from build123d import *

# Parameters (mm, degrees)
F1_DEPTH = 40.2336
F0_R     = 10.16
F2_DEPTH = 15.7734
F3_R     = 3.302


with BuildPart() as f1:
    # F0 (on Front) → F1 (new body)
    with BuildSketch(Plane.XZ):
        with BuildLine():
            ThreePointArc((-46.7830288695, 26.6589681412), (-51.5056559342, 28.027918724), (-56.3930534915, 28.5669708617))
            Line((-56.3930534915, 28.5669708617), (-46.7830288695, 26.6589681412))
        make_face()
        with BuildLine():
            Line((-45.9697033865, -26.3306877774), (-57.2444129947, -28.5744701634))
            ThreePointArc((-57.2444129947, -28.5744701634), (-51.4930580564, -28.0254145609), (-45.9697033865, -26.3306877774))
        make_face()
        with BuildLine():
            Line((-46.7830288695, 26.6589681412), (-56.3930534915, 28.5669708617))
            ThreePointArc((-56.3930534915, 28.5669708617), (-85.6422307581, 0.4256962659), (-57.2444129947, -28.5744701634))
            Line((-57.2444129947, -28.5744701634), (-45.9697033865, -26.3306877774))
            ThreePointArc((-45.9697033865, -26.3306877774), (-33.2614425676, -15.8007621125), (-28.4954018406, 0))
            ThreePointArc((-28.4954018406, 0), (-33.506740117, 16.1642961856), (-46.7830288695, 26.6589681412))
        make_face()
        with BuildLine():
            ThreePointArc((-47.01702871, -10.1519626155), (-71.3571450466, -0.1470537858), (-47.2281253638, 10.3567490075))
            Line((-47.2281253638, 10.3567490075), (-38.5411018406, 10.3567490075))
            Line((-38.5411018406, 10.3567490075), (-38.5411018406, -10.1519626155))
            Line((-38.5411018406, -10.1519626155), (-47.01702871, -10.1519626155))
        make_face(mode=Mode.SUBTRACT)
    extrude(amount=F1_DEPTH)

    # F0 (on Front) → F2 (join)
    with BuildSketch(Plane.XZ):
        with BuildLine():
            Line((12.9274923096, 14.8038646076), (-46.7830288695, 26.6589681412))
            ThreePointArc((-46.7830288695, 26.6589681412), (-33.506740117, 16.1642961856), (-28.4954018406, 0))
            ThreePointArc((-28.4954018406, 0), (-33.2614425676, -15.8007621125), (-45.9697033865, -26.3306877774))
            Line((-45.9697033865, -26.3306877774), (12.9274923096, -14.6095441843))
            ThreePointArc((12.9274923096, -14.6095441843), (19.8690099187, 0.0971602116), (12.9274923096, 14.8038646076))
        make_face()
        with Locations((-3.0954018406, 0)):
            Circle(F0_R, mode=Mode.SUBTRACT)
    extrude(amount=F2_DEPTH)

    # F3
    f3_edges = [f1.edges().sort_by_distance(p)[0] for p in [
        (-57.74775, -40.2336, -28.566971),
    ]]
    fillet(f3_edges, radius=F3_R)


solid = f1.part
Geometry: final body of the model. Coordinates: model frame, mm. A direction names the side the tool comes from. Give positions to 0.01 mm unless a question says otherwise; leave off trailing zeros. Order: outer loops, then holes, each group sorted by start corner. A loop starts at its lowest first (then second) coordinate and runs counter-clockwise, first axis right, second up. Notation, with made-up numbers: (-23.75, 69.25) -> (2.25, 69.25) arc R18 ccw to (2.25, 94.25) -> close; hole circle Ø1 at (14.25, 29). An arc over 180 degrees is marked (long way). Answer as a JSON object with one key per item and string values.
Q1. Section A-A (y = -12). State how many separate pieces and enclosed holes the cut face has, plus the area to 3 significant figures.
Entries:
{"separate pieces": "1", "enclosed holes": "2", "area": "3,380 mm^2"}
Q2. Material intervals for probe 1 along X at (y, z) = (-28, 0); probe 2 along X at (y, z) = (-10, -4); probe 3 along Z at (x, y) = (-57, -35), sorted ascending.
Entries:
{"probe 1": "x = -85.65 to -71.36, -38.54 to -28.5", "probe 2": "x = -85.36 to -70.79, -38.54 to -12.43, 6.24 to 19.42", "probe 3": "z = -28.57 to -14.29, 14.29 to 28.57"}
Q3. Draft query along X for faces 3 (the flat face through (-38.541, -20, 0)), 4 (the flat face through (-14, -15.773, 1)), 5 (the flat face through (-16.93, -7.78, -20.55)). Return one class per face: released by +X, released by -X, zero draft, split by the parting line, or undercut.
Entries:
{"face 3": "undercut", "face 4": "zero draft", "face 5": "released by +X"}
Q4. First-contact query: pin 1 (8 mm diameter, centred on y = -16.5, z = 6.5, fed in from +X); pin 2 (9.5 mm diameter, centred on x = -44.5, y = -15.5, fed in from -Z); pin 3 (10 mm diameter, centred on x = -24.5, y = -10.5, fed in from +Z). Flat tips, straight axial feed; report the tip coordinate or a pass-through.
Entries:
{"pin 1": "stops at x = 19.71", "pin 2": "stops at z = -27.48", "pin 3": "stops at z = 23.23"}
Q5. Access query for faces 1 (the flat face through (-16.51, -7.78, 20.65)), 2 (the flat face through (-43, -20, -10.152)). Directions: +Z, -Z, +X, -X, +Y, -Y. A direction counts if a zero-diameter tool reaches every point of the face in a straight line with its end or side. Return the directions, or none.
Entries:
{"face 1": "+Z, +X, +Y, -Y", "face 2": "+Y, -Y"}
Q6. Section C-C (x = 0). Output: boundary loops of the cut face in (y, z).
Entries:
{"outline": "(-15.77, -17.18) -> (0, -17.18) -> (0, -9.68) -> (-15.77, -9.68) -> close; (-15.77, 9.68) -> (0, 9.68) -> (0, 17.37) -> (-15.77, 17.37) -> close"}
